from build123d import *

# Parameters (mm, degrees)
SKETCH1_W               = 10
SKETCH1_H               = 10
SKETCH1_W_2             = 7
SKETCH1_H_2             = 7
EXTRUDE_THIN1_DEPTH     = 220
CUT_EXTRUDE1_DEPTH      = 221.113607031
CUT_EXTRUDE1_DEPTH_BACK = 221.113607031
SKETCH2_R               = 2.25
FILLET1_R               = 0.2
CUT_EXTRUDE2_REACH      = 222.284
SKETCH5_W               = 5
SKETCH5_H               = 25
BOSS_EXTRUDE3_DEPTH     = 1.5
CHAMFER1_SIZE           = 2


with BuildPart() as part:
    # Sketch1 → Extrude-Thin1 (new body)
    with BuildSketch(Plane(origin=(0, 0, 0), x_dir=(1, 0, 0), z_dir=(0, 1, 0))):
        Rectangle(SKETCH1_W, SKETCH1_H)
        Rectangle(SKETCH1_W_2, SKETCH1_H_2, mode=Mode.SUBTRACT)
    extrude(amount=EXTRUDE_THIN1_DEPTH)

    # Sketch2 → Cut-Extrude1 (cut, two sides: drawn at the far end of the back side and taken through both)
    with BuildSketch(Plane(origin=(0, 0, 0), x_dir=(0, 0, -1), z_dir=(1, 0, 0)).offset(-CUT_EXTRUDE1_DEPTH_BACK)):
        with Locations((0, 215)):
            Circle(SKETCH2_R)
        with Locations(Location((0, 5, 0), (0, 0, 180))):
            Circle(SKETCH2_R)
    extrude(amount=CUT_EXTRUDE1_DEPTH + CUT_EXTRUDE1_DEPTH_BACK, mode=Mode.SUBTRACT)

    # Fillet1
    fillet1_edges = [part.edges().sort_by_distance(p)[0] for p in [
        (-5, 110, -5),
        (5, 110, -5),
        (5, 110, 5),
        (-5, 110, 5),
    ]]
    fillet(fillet1_edges, radius=FILLET1_R)

    # Sketch5 → Cut-Extrude2 (cut, up to next)
    with BuildSketch(Plane(origin=(0, 0, -5), x_dir=(-1, 0, 0), z_dir=(0, 0, -1)), mode=Mode.PRIVATE) as cut_extrude2_sk1:
        with Locations((0, 207.5)):
            Rectangle(SKETCH5_W, SKETCH5_H)
    cut_extrude2_tool1 = extrude(cut_extrude2_sk1.sketch, amount=-CUT_EXTRUDE2_REACH, mode=Mode.PRIVATE) & part.part
    # Sketch5 → Cut-Extrude2 (cut, up to next)
    with BuildSketch(Plane(origin=(0, 0, -5), x_dir=(-1, 0, 0), z_dir=(0, 0, -1)), mode=Mode.PRIVATE) as cut_extrude2_sk2:
        with Locations((0, 12.5)):
            Rectangle(SKETCH5_W, SKETCH5_H)
    cut_extrude2_tool2 = extrude(cut_extrude2_sk2.sketch, amount=-CUT_EXTRUDE2_REACH, mode=Mode.PRIVATE) & part.part
    add(cut_extrude2_tool1.solids().sort_by_distance((0, 207.5, -5))[0], mode=Mode.SUBTRACT)
    add(cut_extrude2_tool2.solids().sort_by_distance((0, 12.5, -5))[0], mode=Mode.SUBTRACT)

    # Sketch5<3> → Boss-Extrude3 (add)
    with BuildSketch(Plane(origin=(0, 0, -5), x_dir=(-1, 0, 0), z_dir=(0, 0, -1))):
        Polygon((4.8, 0), (4.8, 27.5), (-4.8, 27.5), (-4.8, 0), (-2.5, 0), (-2.5, 25), (2.5, 25), (2.5, 0), align=None)
        Polygon((-4.8, 192.5), (4.8, 192.5), (4.8, 220), (2.5, 220), (2.5, 195), (-2.5, 195), (-2.5, 220), (-4.8, 220), align=None)
    extrude(amount=BOSS_EXTRUDE3_DEPTH)

    # Chamfer1
    # the kernel refuses this chamfer: 2 mm, written as the material it adds along each edge
    with BuildSketch(Plane(origin=(-4.8, 27.5, -5), x_dir=(0, 0.9996219169112968, 0.02749587661058694), z_dir=(1, 0, 0))) as chamfer1_piece_1_section:
        Polygon((CHAMFER1_SIZE * 0.999621916911, -CHAMFER1_SIZE * 0.0274958766106), (-CHAMFER1_SIZE * 0.0274958766106, -CHAMFER1_SIZE * 0.999621916911), (0, 0), align=None)
    chamfer1_piece_1 = extrude(amount=9.6, mode=Mode.PRIVATE)
    chamfer1_piece_1 = split(chamfer1_piece_1, bisect_by=Plane(origin=(0, 28.20391822, -6.5), z_dir=(0, 0, 1)), keep=Keep.TOP, mode=Mode.PRIVATE)
    add(chamfer1_piece_1)
    with BuildSketch(Plane(origin=(4.8, 192.5, -5), x_dir=(0, -0.9996219169112968, 0.027495876610586605), z_dir=(-1, 0, 0))) as chamfer1_piece_2_section:
        Polygon((CHAMFER1_SIZE * 0.999621916911, -CHAMFER1_SIZE * 0.0274958766106), (-CHAMFER1_SIZE * 0.0274958766106, -CHAMFER1_SIZE * 0.999621916911), (0, 0), align=None)
    chamfer1_piece_2 = extrude(amount=9.6, mode=Mode.PRIVATE)
    chamfer1_piece_2 = split(chamfer1_piece_2, bisect_by=Plane(origin=(0, 191.79608178, -6.5), z_dir=(0, 0, 1)), keep=Keep.TOP, mode=Mode.PRIVATE)
    add(chamfer1_piece_2)


solid = part.part
For this review, take the finished solid that the model builds, in its own axes (mm). A direction names the side the tool comes from. Round coordinates to 2 decimals unless told otherwise and drop trailing zeros. Write each loop counter-clockwise with the first axis right and the second up, starting at its lowest first coordinate (ties: lowest second). Pieces come first, ordered by that corner, then holes. Notation, with made-up numbers: (-28.5, -9) - (2.5, -9) arc R19 cw to (2.5, 10) - close; hole circle Ø10 at (89.5, 0). An arc over 180 degrees is marked (long way). Use a Markdown table: item, result.
Q1. We need section C-C (z = 0). Give the boundary of the cut face in (x, y), plus the area to 3 significant figures.
Derived:
| item | result |
|---|---|
| outline | (-5, 0) - (-3.5, 0) - (-3.5, 2.75) - (-5, 2.75) - close; (-5, 7.25) - (-3.5, 7.25) - (-3.5, 212.75) - (-5, 212.75) - close; (-5, 217.25) - (-3.5, 217.25) - (-3.5, 220) - (-5, 220) - close; (3.5, 0) - (5, 0) - (5, 2.75) - (3.5, 2.75) - close; (3.5, 7.25) - (5, 7.25) - (5, 212.75) - (3.5, 212.75) - close; (3.5, 217.25) - (5, 217.25) - (5, 220) - (3.5, 220) - close |
| area | 633 mm2 |
Q2. We need section B-B (y = 65). Give the boundary of the cut face in (x, z).
Derived:
| item | result |
|---|---|
| outline | (-5, -4.8) arc R0.2 ccw to (-4.8, -5) - (4.8, -5) arc R0.2 ccw to (5, -4.8) - (5, 4.8) arc R0.2 ccw to (4.8, 5) - (-4.8, 5) arc R0.2 ccw to (-5, 4.8) - close; hole (-3.5, -3.5) - (3.5, -3.5) - (3.5, 3.5) - (-3.5, 3.5) - close |
Q3. Machinability: for faces 1 (the flat face through (0, 108, -3.5)), 2 (the cylindrical face through (-4.26, 217.23, 0.29)), 3 (the flat face through (0, 109, -5)), which of the approach directions +Z, -Z, +X, -X, +Y, -Y give a long, thin tool a straight path to every point of the face, cutting with its end or side? Answer none if there is none.
Derived:
| item | result |
|---|---|
| face 1 | +Y, -Y |
| face 2 | +X, -X |
| face 3 | -Z, +X, -X |
Q4. Wall thickness on line 1 along Y through (x, z) = (-4, 0); line 2 along Z through (x, y) = (-3.8, 215); line 3 along X through (y, z) = (18, 2): over which ranges is each line inside the solid? List them lowest first.
Derived:
| item | result |
|---|---|
| line 1 | y = 0 to 2.75, 7.25 to 212.75, 217.25 to 220 |
| line 2 | z = -6.5 to -2.25, 2.25 to 5 |
| line 3 | x = -5 to -3.5, 3.5 to 5 |
Q5. The part is to be moulded in two halves that separate along Y. For faces 4 (the flat face through (4, 220, 0)), 5 (the cylindrical face through (4.24, 217.23, 0.29)), 6 (the flat face through (-3.5, 108, 0)), 7 (the flat face through (0, 0, 4)), say which applies: pulls with the +Y half, pulls with the -Y half, needs draft (parallel to the pull), parting line crosses it, or undercut.
Derived:
| item | result |
|---|---|
| face 4 | pulls with the +Y half |
| face 5 | undercut |
| face 6 | needs draft |
| face 7 | pulls with the -Y half |
Q6. We need section A-A (y = 5). Give the boundary of the cut face in (x, z).
Derived:
| item | result |
|---|---|
| outline | (-5, -4.8) arc R0.2 ccw to (-4.8, -5) - (-4.8, -6.5) - (-2.5, -6.5) - (-2.5, -3.5) - (-3.5, -3.5) - (-3.5, -2.25) - (-5, -2.25) - close; (-5, 2.25) - (-3.5, 2.25) - (-3.5, 3.5) - (3.5, 3.5) - (3.5, 2.25) - (5, 2.25) - (5, 4.8) arc R0.2 ccw to (4.8, 5) - (-4.8, 5) arc R0.2 ccw to (-5, 4.8) - close; (2.5, -6.5) - (4.8, -6.5) - (4.8, -5) arc R0.2 ccw to (5, -4.8) - (5, -2.25) - (3.5, -2.25) - (3.5, -3.5) - (2.5, -3.5) - close |
Q7. Clearance check with flat-ended pins moving along their axes: pin 1 (3.5 mm diameter, centred on x = 0, z = -4.5, fed in from +Y); pin 2 (0.8 mm diameter, centred on y = 13, z = -5.5, fed in from -X); pin 3 (1.5 mm diameter, centred on x = 1.5, z = -1, fed in from +Y); pin 4 (5 mm diameter, centred on x = 0.5, y = 99, fed in from -Z). State where each tip first meets the part, or that it passes through.
Derived:
| item | result |
|---|---|
| pin 1 | stops at y = 195 |
| pin 2 | stops at x = -4.8 |
| pin 3 | passes through |
| pin 4 | stops at z = -5 |
